from build123d import *

# Parameters (mm, degrees)
BOSS_EXTRUDE1_DEPTH = 1.5
SKETCH2_R           = 3
SKETCH2_R_2         = 1.35
SKETCH2_R_3         = 1
CUT_EXTRUDE1_DEPTH  = 25.182451908


with BuildPart() as part:
    # Sketch1 → Boss-Extrude1 (new body)
    with BuildSketch(Plane.XY):
        with BuildLine():
            Line((-3.352285907, -12.464521672), (2.647714093, -12.464521672))
            Line((2.647714093, -12.464521672), (2.647714093, -15.928650375))
            ThreePointArc((2.647714093, -15.928650375), (15.091360711, -6.367255259), (14.403401907, 9.310478328))
            Line((14.403401907, 9.310478328), (13.537376503, 8.810478328))
            ThreePointArc((13.537376503, 8.810478328), (-0.319029957, 16.810478328), (-14.175436418, 8.810478328))
            Line((-14.175436418, 8.810478328), (-15.041461822, 9.310478328))
            ThreePointArc((-15.041461822, 9.310478328), (-15.743655386, -6.336614115), (-3.352285907, -15.916725812))
            Line((-3.352285907, -15.916725812), (-3.352285907, -12.464521672))
        make_face()
    extrude(amount=BOSS_EXTRUDE1_DEPTH)

    # Sketch2 → Cut-Extrude1 (cut, through all)
    with BuildSketch(Plane.XY.offset(1.5)):
        with Locations((-10.102285907, -5.464521672)):
            Circle(SKETCH2_R)
        with Locations(Location((9.397714093, -5.464521672, 0), (0, 0, 180))):
            Circle(SKETCH2_R)
        with Locations((-12.977285907, 5.060478328)):
            Circle(SKETCH2_R_2)
        with Locations(Location((12.272714093, 5.060478328, 0), (0, 0, 180))):
            Circle(SKETCH2_R_2)
        with Locations((-4.652285907, -6.939521672)):
            Circle(SKETCH2_R_3)
        with Locations(Location((3.947714093, -6.939521672, 0), (0, 0, 180))):
            Circle(SKETCH2_R_3)
    extrude(amount=-CUT_EXTRUDE1_DEPTH, mode=Mode.SUBTRACT)


solid = part.part
Could you check a few things on this model? Use its own coordinates, in mm. A direction names the side the tool comes from. Give positions to 0.01 mm unless a question says otherwise; leave off trailing zeros. Loops run counter-clockwise (first coordinate to the right, second up) from the corner with the lowest first, then second, coordinate; pieces in that order, holes last. Notation, with made-up numbers: M 0,76 L 13,76 A10 ccw 13,86 Z; hole C -27,50.25 d1. An arc over 180 degrees is marked long. Answer as a JSON object with one key per item and string values.
Q1. For faces 4 (the flat face through (13.976, 9.064, 0.74)), 5 (the flat face through (2.648, -14, 1)), 6 (the cylindrical face through (-3.729, -7.323, 0.76)), which set-ups out of +Z, -Z, +X, -X, +Y, -Y let a thin tool reach every point of the face, with its end or its side?
Values found:
{"face 4": "+Z, -Z, +Y", "face 5": "+Z, -Z, -Y", "face 6": "+Z, -Z"}
Q2. Suppose I cut it at B-B, the plane y = -5. List the corners of the cut face in (x, z) for me, plus the area to 3 significant figures.
Values found:
{"outline": "M -16.3,0 L -13.07,0 L -13.07,1.5 L -16.3,1.5 Z; M -7.14,0 L 6.43,0 L 6.43,1.5 L -7.14,1.5 Z; M 12.36,0 L 15.66,0 L 15.66,1.5 L 12.36,1.5 Z", "area": "30.1 mm²"}
Q3. If I drill on probe 1 along X at (y, z) = (-6.5, 0.8); probe 2 along X at (y, z) = (-4, 0.15); probe 3 along X at (y, z) = (5.5, 1.3), over which ranges is the centre line in solid material (lowest first)? Write a range as [from, to].
Values found:
{"probe 1": "x = [-15.67, -12.92], [-7.29, -5.55], [-3.75, 3.05], [4.85, 6.58], [12.21, 15.03]", "probe 2": "x = [-16.62, -12.72], [-7.48, 6.78], [12.02, 15.99]", "probe 3": "x = [-16.66, -14.25], [-11.7, 11], [13.55, 16.02]"}
Q4. Suppose I cut it at A-A, the plane x = 7.5. List the corners of the cut face in (y, z) for me.
Values found:
{"outline": "M -14.28,0 L -7.79,0 L -7.79,1.5 L -14.28,1.5 Z; M -3.14,0 L 14.77,0 L 14.77,1.5 L -3.14,1.5 Z"}
Q5. Suppose I cut it at D-D, the plane z = 0.3. List the corners of the cut face in (x, y) for me, plus the area to 3 significant figures.
Values found:
{"outline": "M -15.04,9.31 A17 ccw -3.35,-15.92 L -3.35,-12.46 L 2.65,-12.46 L 2.65,-15.93 A17 ccw 14.4,9.31 L 13.54,8.81 A16 ccw -14.18,8.81 Z; hole C -12.98,5.06 d2.7; hole C -10.1,-5.46 d6; hole C -4.65,-6.94 d2; hole C 3.95,-6.94 d2; hole C 9.4,-5.46 d6; hole C 12.27,5.06 d2.7", "area": "777 mm²"}
Q6. If we mould it in two halves opening along Y, with no side actions, what happens to faces 1 (the cylindrical face through (14.994, -6.574, 0.74)), 2 (the flat face through (-1, 1, 1.5)), 3 (the cylindrical face through (4.7, -7.6, 0.8))? For each: pulls with the +Y half, pulls with the -Y half, needs draft (parallel to the pull), parting line crosses it, or undercut.
Values found:
{"face 1": "parting line crosses it", "face 2": "needs draft", "face 3": "undercut"}
Q7. Suppose I cut it at C-C, the plane y = -14. List the corners of the cut face in (x, z) for me.
Values found:
{"outline": "M -8.66,0 L -3.35,0 L -3.35,1.5 L -8.66,1.5 Z; M 2.65,0 L 8.03,0 L 8.03,1.5 L 2.65,1.5 Z"}
